Model file for the job. Use its own axes, mm. Round coordinates to 2 decimals unless told otherwise and drop trailing zeros. Loops run counter-clockwise (first coordinate to the right, second up) from the corner with the lowest first, then second, coordinate; pieces in that order, holes last.
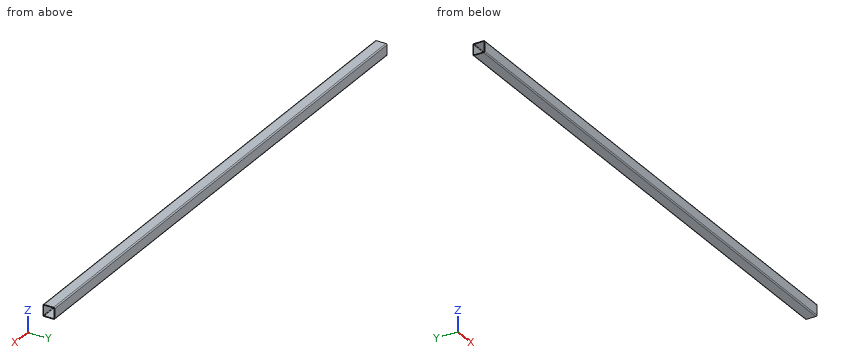
from build123d import *

# Parameters (mm, degrees)
F0_W     = 50.8
F0_H     = 50.8
F1_DEPTH = 1168.4
F2_T     = -3.175
F3_R     = 4.7625
F4_R     = 2.38125


with BuildPart() as f1:
    # F0 (on Right) → F1 (new body, symmetric)
    with BuildSketch(Plane.YZ):
        Rectangle(F0_W, F0_H)
    extrude(amount=F1_DEPTH, both=True)

    # F2
    f2_openings = [f1.faces().sort_by_distance(p)[0] for p in [
        (1168.4, 0, 0),
        (-1168.4, 0, 0),
    ]]
    offset(amount=F2_T, openings=f2_openings)

    # F3
    f3_edges = [f1.edges().sort_by_distance(p)[0] for p in [
        (0, 25.4, 25.4),
        (0, -25.4, 25.4),
        (0, 25.4, -25.4),
        (0, -25.4, -25.4),
    ]]
    fillet(f3_edges, radius=F3_R)

    # F4
    f4_edges = [f1.edges().sort_by_distance(p)[0] for p in [
        (0, -22.225, 22.225),
        (0, -22.225, -22.225),
        (0, 22.225, -22.225),
        (0, 22.225, 22.225),
    ]]
    fillet(f4_edges, radius=F4_R)


solid = f1.part
Q1. Slice it at A-A on x = -934. Give the cut face in (y, z) (1 decimal), plus the area to 3 significant figures.
Q2. Probe line 1 (Z direction, x = -956.5, y = -6) (3 decimals); line 2 (Y direction, x = 103.5, z = -22). List the from-to ranges inside material, lowest first.
Q3. Slice it at B-B on z = -4. Give the cut face in (x, y) (3 decimals).
Q4. Flat gauge pin, fed straight in: P1, Ø12, axis at y = 0.5, z = 14, coming from the +X side. Where does the tip first touch, or does it go through?
Reply:
1. outline: (-25.4, -20.6) arc R4.8 ccw to (-20.6, -25.4) - (20.6, -25.4) arc R4.8 ccw to (25.4, -20.6) - (25.4, 20.6) arc R4.8 ccw to (20.6, 25.4) - (-20.6, 25.4) arc R4.8 ccw to (-25.4, 20.6) - close; hole (-22.2, -19.8) arc R2.4 ccw to (-19.8, -22.2) - (19.8, -22.2) arc R2.4 ccw to (22.2, -19.8) - (22.2, 19.8) arc R2.4 ccw to (19.8, 22.2) - (-19.8, 22.2) arc R2.4 ccw to (-22.2, 19.8) - close
1. area: 590 mm2
2. line 1: z = -25.4 to -22.225, 22.225 to 25.4
2. line 2: y = -25.2 to -20.85, 20.85 to 25.2
3. outline: (-1168.4, -25.4) - (1168.4, -25.4) - (1168.4, -22.225) - (-1168.4, -22.225) - close; (-1168.4, 22.225) - (1168.4, 22.225) - (1168.4, 25.4) - (-1168.4, 25.4) - close
4. P1: passes through
